For this review, take the finished solid that the model builds, in its own axes (mm). Face numbers are marked on the shaded views. A direction names the side the tool comes from. Give positions to 0.01 mm unless a question says otherwise; leave off trailing zeros. Write each loop counter-clockwise with the first axis right and the second up, starting at its lowest first coordinate (ties: lowest second). Pieces come first, ordered by that corner, then holes. Notation, with made-up numbers: M 23.5,1.5 L 57.5,1.5 A6 cw 57.5,12.5 Z; hole C 14,86.5 d10. An arc over 180 degrees is marked long. One line per item, written item: value. Start each with the question number.
Item 1: Consider section C-C, the plane y = 0. Write out the cut boundary in (x, z).
Item 2: Consider section D-D, the plane x = -180. Write out the cut boundary in (y, z).
Item 3: Tool access review of the marked faces 4, 5, 6 and 7: name each direction out of +Z, -Z, +X, -X, +Y, -Y from which nothing blocks a thin tool from reaching the whole face with its end or side.
Item 4: Consider section A-A, the plane x = -136.5. Write out the cut boundary in (y, z).
Item 5: To check wall thickness, follow probe 1 along X at (y, z) = (16.5, 2); probe 2 along Y at (x, z) = (-141, -3.5). State the ranges of each line that lie inside material, in increasing order.
Item 6: Consider section B-B, the plane z = 0. Write out the cut boundary in (x, y).
Item 7: Clearance check with flat-ended pins moving along their axes: pin 1 Ø1.5 at (x, z) = (-128.5, 15.5) entering from -Y; pin 2 Ø3 at (x, y) = (-212.5, 13) entering from +Z; pin 3 Ø12 at (x, y) = (-177, 6.5) entering from +Z (3 decimals). State where each tip first meets the part, or that it passes through.
Item 8: Mouldability with a two-part tool opening along X and no side actions: class the marked faces 1, 2 and 3 as released by +X, released by -X, zero draft, split by the parting line, or undercut.
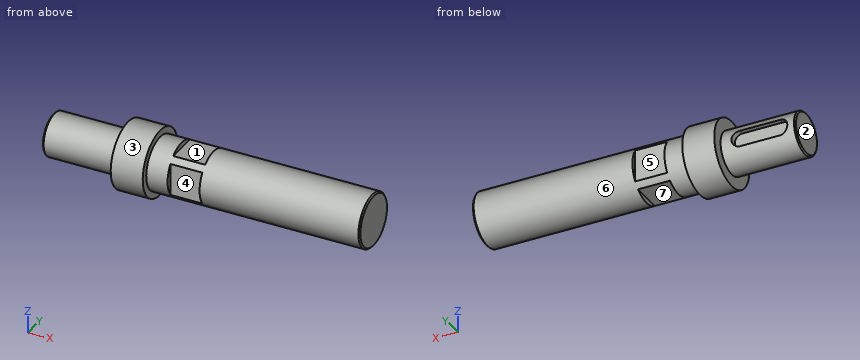
```python
from build123d import *

# Parameters (mm, degrees)
SKETCH_2_OUTSIDE_W   = 102.04
SKETCH_2_OUTSIDE_H   = 102.04
SKETCH_2_OUTSIDE_W_2 = 32
SKETCH_2_OUTSIDE_H_2 = 32
CUT_EXTRUDE_1_DEPTH  = 24
CUT_EXTRUDE_2_DEPTH  = 5


with BuildPart() as part:
    # Эскиз1 → Повернуть1 (revolve)
    with BuildSketch(Plane.XY, mode=Mode.PRIVATE) as revolve_1_sk:
        Polygon((0, 0), (0, 19), (-1, 20), (-160, 20), (-160, 25), (-184, 25), (-184, 16), (-239, 16), (-240, 15), (-240, 0), align=None)
    revolve(revolve_1_sk.sketch.rotate(Axis((-178.322580645, 0, 0), (1, 0, 0)), 90), axis=Axis((-178.322580645, 0, 0), (1, 0, 0)))

    # Эскиз2 outside → Вырез-Вытянуть1 (cut)
    with BuildSketch(Plane(origin=(-144, 0, 0), x_dir=(0, 0, -1), z_dir=(1, 0, 0))):
        Rectangle(SKETCH_2_OUTSIDE_W, SKETCH_2_OUTSIDE_H)
        Rectangle(SKETCH_2_OUTSIDE_W_2, SKETCH_2_OUTSIDE_H_2, mode=Mode.SUBTRACT)
    extrude(amount=CUT_EXTRUDE_1_DEPTH, mode=Mode.SUBTRACT)

    # Эскиз3 → Вырез-Вытянуть2 (cut)
    with BuildSketch(Plane(origin=(0, 16, 0), x_dir=(1, 0, 0), z_dir=(0, 1, 0))):
        with BuildLine():
            Line((-228, 6), (-198, 6))
            ThreePointArc((-198, 6), (-192, 0), (-198, -6))
            Line((-198, -6), (-228, -6))
            ThreePointArc((-228, -6), (-234, 0), (-228, 6))
        make_face()
    extrude(amount=-CUT_EXTRUDE_2_DEPTH, mode=Mode.SUBTRACT)


solid = part.part
```
Model answer:
1. outline: M -240,-15 L -239,-16 L -184,-16 L -184,-25 L -160,-25 L -160,-20 L -144,-20 L -144,-16 L -120,-16 L -120,-20 L -1,-20 L 0,-19 L 0,19 L -1,20 L -120,20 L -120,16 L -144,16 L -144,20 L -160,20 L -160,25 L -184,25 L -184,16 L -239,16 L -240,15 Z
2. outline: C 0,0 d50
3. face 4: +Z, -Z, -Y
3. face 5: +Z, -Z, +Y
3. face 6: +X
3. face 7: -Z, +Y, -Y
4. outline: M -16,-12 A20 ccw -12,-16 L 12,-16 A20 ccw 16,-12 L 16,12 A20 ccw 12,16 L -12,16 A20 ccw -16,12 Z
5. probe 1: x = -184 to -144, -120 to 0
5. probe 2: y = -16 to 16
6. outline: M -240,-15 L -239,-16 L -184,-16 L -184,-25 L -160,-25 L -160,-20 L -144,-20 L -144,-16 L -120,-16 L -120,-20 L -1,-20 L 0,-19 L 0,19 L -1,20 L -120,20 L -120,16 L -144,16 L -144,20 L -160,20 L -160,25 L -184,25 L -184,16 L -192,16 L -192,11 L -234,11 L -234,16 L -239,16 L -240,15 Z
7. pin 1: stops at y = -13.51
7. pin 2: stops at z = 11.12
7. pin 3: stops at z = 24.995
8. face 1: undercut
8. face 2: released by -X
8. face 3: zero draft
